For this review, take the finished solid that the model builds, in its own axes (mm). A direction names the side the tool comes from. Give positions to 0.01 mm unless a question says otherwise; leave off trailing zeros. Order: outer loops, then holes, each group sorted by start corner. A loop starts at its lowest first (then second) coordinate and runs counter-clockwise, first axis right, second up. Notation, with made-up numbers: (-28.5, 59) - (6.5, 59) arc R18 cw to (6.5, 84) - close; hole circle Ø6 at (-20, -33.75). An arc over 180 degrees is marked (long way). Use a Markdown table: item, result. Add a question column.
1) Mouldability with a two-part tool opening along Z and no side actions: class faces 6 (the face through (-10.97, 10.76, 14.34)), 7 (the face through (-7, 3, 14)), 8 (the face through (10, 10, -12)) as released by +Z, released by -Z, zero draft, split by the parting line, or undercut.
2) We need section C-C on x = 0. Write out the cut boundary in (y, z), then the cut area to 3 significant figures.
3) We need section B-B on y = 3.75. Write out the cut boundary in (x, z), then the cut area to 3 significant figures.
4) Wall thickness on L1, parallel to X at y = 1.5, z = 0; L2, parallel to Z at x = -11.55, y = 12; L3, parallel to Z at x = 9.2, y = 12: over which ranges is each line inside the solid? List them lowest first.
5) Machinability: for faces 1 (the face through (-7, 3, -15)), 2 (the face through (9.014, 8.778, 6.077)), 3 (the face through (10, 4, 13)), 4 (the face through (-3, 2, 0)), 5 (the face through (-11.028, 17.715, 12.301)), which of the approach directions +Z, -Z, +X, -X, +Y, -Y give a long, thin tool a straight path to every point of the face, cutting with its end or side? Answer none if there is none.
6) We need section D-D on z = -5. Write out the cut boundary in (x, y).
7) We need section A-A on x = -10. Write out the cut boundary in (y, z), then the cut area to 3 significant figures.
8) Clearance check with flat-ended pins moving along their axes: P1, Ø5.5, axis at y = 14.5, z = 15.5, coming from the +X side; P2, Ø6, axis at y = 12, z = 6.5, coming from the -X side; P3, Ø12, axis at x = -2.5, z = 12.5, coming from the +Y side. State where each tip first meets the part, or that it passes through.
Autodesk Inventor part; units mm, degrees
ref_plane "YZ Plane" through (0, 0, 0) normal (1, 0, 0) x (0, 1, 0)
ref_plane "XZ Plane" through (0, 0, 0) normal (0, 1, 0) x (-1, 0, 0)
ref_plane "XY Plane" through (0, 0, 0) normal (0, 0, 1) x (1, 0, 0)
sketch "Sketch1" plane through (0, 0, 0) normal (0, 1, 0) x (-1, 0, 0)
  line L0 (15.4, 0) -> (-15.4, 0)
  line L1 (0, -23.8) -> (0, 23.8)
  line L2 (11, 17) -> (-11, 17)
  line L3 (-11, 17) -> (-11, -17)
  line L4 (-11, -17) -> (11, -17)
  line L5 (11, -17) -> (11, 17)
  point P0 (0, 0)
  dimension "d0" = 22
  dimension "d1" = 34
extrude "Extrusion1" add sketch "Sketch1" along normal blind 18
sketch "Sketch2" plane through (0, 18, 0) normal (0, 1, 0) x (1, 0, 0)
  line L0 (-11, -12) -> (8, -12)
  line L1 (8, -12) -> (8, 12)
  line L2 (8, 12) -> (-11, 12)
  line L3 (-11, 12) -> (-11, -12)
  line L4 (-11, -17) -> (11, -17)
  line L5 (11, -17) -> (11, 17)
  line L6 (11, 17) -> (-11, 17)
  line L7 (-11, 17) -> (-11, -17)
  line L8 (-15.4, 0) -> (15.4, 0)
  point P0 (0, 0)
  dimension "d5" = 24
  dimension "d6" = 3
extrude "Extrusion2" cut sketch "Sketch2" against normal blind 16 contours L3 L8 L1 L0 | L3 L2 L1 L8
sketch "Sketch3" plane through (-11, 0, 17) normal (0, 0, 1) x (1, 0, 0)
  line L0 (4, 18) -> (19, 18)
  line L1 (19, 18) -> (19, 2)
  line L2 (19, 2) -> (4, 2)
  line L3 (4, 2) -> (4, 18)
  line L4 (0, 18) -> (22, 18)
  line L5 (0, 0) -> (0, 18)
  line L6 (22, 0) -> (22, 18)
  line L7 (0, 0) -> (22, 0)
  point P0 (11, 0)
  dimension "d9" = 4
  dimension "d10" = 3
  dimension "d11" = 2
extrude "Extrusion3" cut sketch "Sketch3" against normal through all contours L0 L1 L2 L3
sketch "Sketch6" plane through (0, 2, 0) normal (0, 1, 0) x (1, 0, 0)
  line L0 (-11, 12) -> (-7, 12)
  line L1 (-11, -12) -> (-11, 12)
  line L2 (-7, -12) -> (-11, -12)
  line L3 (-7, -17) -> (-7, -12)
  line L4 (8, -17) -> (-7, -17)
  line L5 (-7, 17) -> (8, 17)
  line L6 (-7, 12) -> (-7, 17)
  line L7 (-15.4, 0) -> (15.4, 0)
  line L8 (0, 23.8) -> (0, -23.8)
  line L9 (8, -17) -> (8, 17)
  point P0 (0, 0)
  point P1 (0, 0)
  point P2 (0, 6)
  point P3 (0, -6)
  point P4 (-6, 0)
  dimension "d15" = 6
  dimension "d16" = 6
  dimension "d18" = 6
hole "Hole1" at (0, 2, -6) at (0, 2, 0) at (0, 2, 6) at (-6, 2, 0) direction (0, -1, 0) diameter 3 end through all
sketch "Sketch8" plane through (11, 0, 17) normal (1, 0, 0) x (0, 0, -1)
  line L0 (0, 0) -> (34, 0)
  line L1 (34, 0) -> (34, 18)
  line L2 (0, 18) -> (34, 18)
  line L3 (0, 0) -> (0, 18)
  line L4 (29, 2) -> (29, 18)
  line L5 (5, 18) -> (5, 2)
  line L6 (29, 2) -> (5, 2)
  point P0 (17, 0)
  point P1 (0, 2)
  point P2 (34, 2)
  point P3 (23.5, 12)
  point P4 (10.5, 12)
  dimension "d28" = 5.5
  dimension "d29" = 5.5
  dimension "d30" = 6
  dimension "d31" = 6
hole "Hole2" at (11, 12, -6.5) at (11, 12, 6.5) direction (-1, 0, 0) diameter 4.5 end through all
sketch "Sketch12" plane through (0, 18, 0) normal (0, 1, 0) x (1, 0, 0)
  line L0 (8, 17) -> (8, -17)
  line L1 (8, -17) -> (11, -17)
  line L2 (11, -17) -> (11, 17)
  line L3 (11, 17) -> (8, 17)
  line L4 (8, -17) -> (11, -17)
  line L5 (11, -17) -> (11, -12)
  line L6 (11, -12) -> (8, -12)
  line L7 (8, -12) -> (8, -17)
  line L8 (8, 17) -> (11, 17)
  line L9 (11, 17) -> (11, 12)
  line L10 (11, 12) -> (8, 12)
  line L11 (8, 12) -> (8, 17)
  line L12 (-7, -17) -> (-7, -12)
  line L13 (-7, -12) -> (-11, -12)
  line L14 (-11, -12) -> (-11, -17)
  line L15 (-11, -17) -> (-7, -17)
  line L16 (-7, 12) -> (-7, 17)
  line L17 (-7, 17) -> (-11, 17)
  line L18 (-11, 17) -> (-11, 12)
  line L19 (-11, 12) -> (-7, 12)
  point P0 (0, 0)
extrude "Extrusion5" cut sketch "Sketch12" against normal blind 16 contours L3 L2 L10 L0 | L6 L2 L1 L0
sketch "Sketch17" plane through (-11, 0, -17) normal (-1, 0, 0) x (0, 0, 1)
  line L0 (29, 18) -> (29, 2)
  line L1 (29, 2) -> (5, 2)
  line L2 (5, 2) -> (5, 18)
  line L3 (0, 18) -> (5, 18)
  line L4 (0, 0) -> (0, 18)
  line L5 (0, 0) -> (34, 0)
  line L6 (34, 0) -> (34, 18)
  line L7 (29, 18) -> (34, 18)
  line L8 (34, 0) -> (0, 0)
  line L9 (29, 18) -> (29, 2)
  line L10 (34, 0) -> (29, 0)
  line L11 (29, 0) -> (29, 18)
  line L12 (29, 18) -> (34, 18)
  line L13 (34, 18) -> (34, 0)
  line L14 (0, 18) -> (5, 18)
  line L15 (0, 0) -> (5, 0)
  line L16 (5, 0) -> (5, 18)
  line L17 (5, 18) -> (0, 18)
  line L18 (0, 18) -> (0, 0)
  line L19 (0, 2) -> (5, 2)
  line L20 (34, 0) -> (0, 0)
  line L21 (0, 0) -> (0, 2)
  line L22 (0, 2) -> (34, 2)
  line L23 (34, 2) -> (34, 0)
  point P0 (17, 0)
extrude "Extrusion6" add sketch "Sketch17" along normal blind 2
sketch "Sketch19" plane through (8, 18, -12) normal (-1, 0, 0) x (0, 0, 1)
  circle A0 centre (18.5, -6) radius 2.25
  circle A1 centre (5.5, -6) radius 2.25
  line L0 (24, -16) -> (24, 0)
  line L1 (0, 0) -> (24, 0)
  line L2 (0, 0) -> (0, -16)
  line L3 (24, -16) -> (0, -16)
  point P0 (12, -18)
hole "Hole4" at (8, 12, 6.5) at (8, 12, -6.5) direction (1, 0, 0) diameter 6.5 depth 2
fillet "Fillet9" radius 6 2 edges at (9.5, 18, -12) (9.5, 18, 12)
fillet "Fillet10" radius 5 4 edges at (9.5, 2, 12) (9.5, 2, -12) (11, 1, 17) (11, 1, -17)
sketch "Sketch20" plane through (-13, 0, -17) normal (-1, 0, 0) x (0, 0, 1)
  line L0 (0, 0) -> (34, 0)
  line L1 (34, 0) -> (34, 18)
  line L2 (34, 18) -> (29, 18)
  line L3 (29, 18) -> (29, 2)
  line L4 (29, 2) -> (5, 2)
  line L5 (5, 2) -> (5, 18)
  line L6 (5, 18) -> (0, 18)
  line L7 (0, 18) -> (0, 0)
  point P0 (17, 0)
  point P1 (2.5, 12)
  point P2 (31.5, 12)
  dimension "d85" = 6
  dimension "d86" = 2.5
  dimension "d87" = 2.5
  dimension "d88" = 6
hole "Hole5" at (-13, 12, -14.5) at (-13, 12, 14.5) direction (1, 0, 0) diameter 2.5 end through all
sketch "Sketch21" plane through (-7, 2, 17) normal (0, 0, 1) x (1, 0, 0)
  line L0 (-2, 16) -> (0, 16)
  line L1 (0, 16) -> (0, 0)
  line L2 (0, 0) -> (-2, 0)
  line L3 (-2, 0) -> (-2, 16)
  line L4 (13, 0) -> (13, -2)
  line L5 (13, 0) -> (0, 0)
  line L6 (0, 0) -> (0, 16)
  line L7 (0, 16) -> (-6, 16)
  line L8 (-6, -2) -> (-6, 16)
  line L9 (-6, -2) -> (13, -2)
  line L10 (13, 0) -> (0, 0)
  line L11 (0, 16) -> (-6, 16)
  line L12 (0, 0) -> (0, 16)
  point P0 (7, -2)
  dimension "d96" = 4
extrude "Extrusion7" cut sketch "Sketch21" against normal through all contours L0 L1 L2 L3
fillet "Fillet11" radius 5 2 edges at (-9, 2, 14.5) (-9, 2, -14.5)
fillet "Fillet12" radius 1 4 edges at (-11, 18, 17) (-11, 18, 12) (-11, 18, -12) (-11, 18, -17)
properties part number "bracket"
Checked values:
| question | item | result |
|---|---|---|
| 1 | face 6 | undercut |
| 1 | face 7 | zero draft |
| 1 | face 8 | released by -Z |
| 2 | outline | (0, -17) - (2, -17) - (2, -7.5) - (0, -7.5) - close; (0, -4.5) - (2, -4.5) - (2, -1.5) - (0, -1.5) - close; (0, 1.5) - (2, 1.5) - (2, 4.5) - (0, 4.5) - close; (0, 7.5) - (2, 7.5) - (2, 17) - (0, 17) - close |
| 2 | area | 50.0 mm² |
| 3 | outline | (-13, -17) - (-7.8, -17) - (-7.8, -12) - (-13, -12) - close; (-13, 12) - (-7.8, 12) - (-7.8, 17) - (-13, 17) - close; (8, -13.2) - (10.85, -13.2) arc R5 ccw to (11, -12) - (11, 12) arc R5 ccw to (10.85, 13.2) - (8, 13.2) - close |
| 3 | area | 131 mm² |
| 4 | L1 | -13 to -7.5, -4.5 to -1.5, 1.5 to 11 |
| 4 | L2 | -17 to -15.75, -13.25 to -12, 12 to 13.25, 15.75 to 17 |
| 4 | L3 | -12 to -9.75, -3.25 to 3.25, 9.75 to 12 |
| 5 | face 1 | +Z, -Z, +Y |
| 5 | face 2 | -X |
| 5 | face 3 | +Z, +X, +Y |
| 5 | face 4 | +Y |
| 5 | face 5 | +X, -X, +Y |
| 6 | outline | (-13, 0) - (-1.12, 0) - (-1.12, 2) - (-13, 2) - close; (1.12, 0) - (11, 0) - (11, 10.32) - (10, 10.32) - (10, 9.12) - (8, 9.12) - (8, 2) - (1.12, 2) - close; (8, 14.88) - (10, 14.88) - (10, 13.68) - (11, 13.68) - (11, 18) - (8, 18) - close |
| 7 | outline | (0, -17) - (17, -17) arc R1 ccw to (18, -16) - (18, -13) arc R1 ccw to (17, -12) - (2, -12) - (2, 12) - (17, 12) arc R1 ccw to (18, 13) - (18, 16) arc R1 ccw to (17, 17) - (0, 17) - close; hole circle Ø2.5 at (12, -14.5); hole circle Ø2.5 at (12, 14.5) |
| 7 | area | 217 mm² |
| 8 | P1 | x = -9 |
| 8 | P2 | x = 10 |
| 8 | P3 | y = 4.82 |
